CAD build for the part. Positions are in the model's coordinates, mm. A direction names the side the tool comes from. Round coordinates to 2 decimals unless told otherwise and drop trailing zeros. Order: outer loops, then holes, each group sorted by start corner. A loop starts at its lowest first (then second) coordinate and runs counter-clockwise, first axis right, second up. Notation, with made-up numbers: M 63,47 L 113,47 A33 cw 113,81 Z; hole C 9,-10.75 d6. An arc over 180 degrees is marked long. Put each result on its own line as item: value.
```python
from build123d import *

# Parameters (mm, degrees)
F0_W     = 81.7349255085
F0_H     = 55.1976133138
F1_DEPTH = 54.61
F2_W     = 16.1877609789
F2_H     = 56.2591040507
F6_R     = 5.08
F7_SIZE  = 5.08


with BuildPart() as f1:
    # F0 (on Front) → F1 (new body, symmetric)
    with BuildSketch(Plane.XZ):
        with Locations((1.3268664479, 0.9260410443)):
            Rectangle(F0_W, F0_H)
    extrude(amount=F1_DEPTH, both=True)

    # F2 (on Front) → F3 (revolve)
    with BuildSketch(Plane.XZ):
        with Locations((-8.0938804895, 41.5281313471)):
            Rectangle(F2_W, F2_H)
    revolve(axis=Axis((0, 0, 41.5281313471), (0, 0, -1)))

    # F4 (on Front) → F5 (revolve)
    with BuildSketch(Plane.XZ):
        with BuildLine():
            Line((0, 57.0264922878), (0, 118.6706257561))
            ThreePointArc((0, 118.6706257561), (-30.8220667341, 87.8485590219), (0, 57.0264922878))
        make_face()
    revolve(axis=Axis((0, 0, 87.8485590219), (0, 0, -1)))

    # F6
    f6_edges = [f1.edges().sort_by_distance(p)[0] for p in [
        (1.326866, -54.61, 28.524848),
        (42.194329, 0, 28.524848),
        (1.326866, 54.61, 28.524848),
        (-39.540596, 0, 28.524848),
    ]]
    fillet(f6_edges, radius=F6_R)

    # F7
    f7_edges = [f1.edges().sort_by_distance(p)[0] for p in [
        (16.187761, 0, 28.524848),
    ]]
    chamfer(f7_edges, length=F7_SIZE)


solid = f1.part
```
Item 1: Tool access for faces 4 (the flat face through (1, -54.61, -1)), 5 (the conical face through (13.04, 10, 33.36)): list every direction of +Z, -Z, +X, -X, +Y, -Y with a clear straight run to the whole face (end or side of a thin tool).
Answers below:
face 4: +Z, -Z, +X, -X, -Y
face 5: none
Item 2: Band-saw the part on C-C on y = -24. Give the cut face in (x, z), and give its area (3 significant figures).
Answers below:
outline: M -39.54,-26.67 L 42.19,-26.67 L 42.19,23.44 A5.08 ccw 37.11,28.52 L -34.46,28.52 A5.08 ccw -39.54,23.44 Z; C 0,87.85 d38.68
area: 5,680 mm²
Item 3: Pin check, flat tips, straight feed: P1, Ø8, axis at x = 25.5, z = 100.5, coming from the +Y side; P2, Ø2, axis at x = 11.5, z = 52, coming from the -Y side; P3, Ø1.5, axis at x = 22, z = 81.5, coming from the +Y side. Stop position of each tip, or through.
Answers below:
P1: y = 18.75
P2: y = -12.32
P3: y = 21.44
Item 4: Band-saw the part on D-D on x = 0. Give the cut face in (y, z), and give its area (4 significant figures).
Answers below:
outline: M -54.61,-26.67 L 54.61,-26.67 L 54.61,23.44 A5.08 ccw 49.53,28.52 L 21.27,28.52 L 16.19,33.6 L 16.19,61.62 A30.82 ccw long -16.19,61.62 L -16.19,33.6 L -21.27,28.52 L -49.53,28.52 A5.08 ccw -54.61,23.44 Z
area: 10,000 mm²
Item 5: Probe line 1 along Z through (x, y) = (-32.5, 44.5); line 2 along Z through (x, y) = (-16, -10.5); line 3 along Z through (x, y) = (14, -9). List the from-to ranges inside material, lowest first. Write a range as [from, to].
Answers below:
line 1: [-26.67, 28.52]
line 2: [-26.67, 30.65], [63.69, 112.01]
line 3: [-26.67, 33.15], [61.91, 113.79]
Item 6: Band-saw the part on B-B on x = 33.5. Give the cut face in (y, z), and give its area (3 significant figures).
Answers below:
outline: M -54.61,-26.67 L 54.61,-26.67 L 54.61,23.44 A5.08 ccw 49.53,28.52 L -49.53,28.52 A5.08 ccw -54.61,23.44 Z
area: 6,020 mm²
Item 7: Band-saw the part on A-A on y = 0. Give the cut face in (x, z).
Answers below:
outline: M -39.54,-26.67 L 42.19,-26.67 L 42.19,23.44 A5.08 ccw 37.11,28.52 L 21.27,28.52 L 16.19,33.6 L 16.19,61.62 A30.82 ccw long -16.19,61.62 L -16.19,33.6 L -21.27,28.52 L -34.46,28.52 A5.08 ccw -39.54,23.44 Z
Item 8: Mould opens along Z. For faces 1 (the flat face through (1, -23, 28.525)), 2 (the flat face through (42.194, -1, -2)), 3 (the cylindrical face through (1.9, -53.08, 27.08)) say: pulls with the +Z half, pulls with the -Z half, needs draft (parallel to the pull), parting line crosses it, or undercut.
Answers below:
face 1: undercut
face 2: needs draft
face 3: pulls with the +Z half
